```python
from build123d import *

# Parameters (mm, degrees)
F0_W     = 3
F0_H     = 12
F0_W_2   = 7
F0_H_2   = 1
F1_DEPTH = 150
F3_D     = 4.4
F3_DEPTH = 10.4
F3_TIP   = 1.3218933619
F4_SIZE  = 19.99999
F6_DEPTH = 8


# Not quite as in the source:
# - a fillet or chamfer is up to 0.001 mm smaller than in the source, because OpenCascade refuses the exact size


with BuildPart() as f1:
    # F0 (on Front) → F1 (new body)
    with BuildSketch(Plane.XZ):
        with Locations((-8.5, 8)):
            Rectangle(F0_W, F0_H)
        Polygon((-10, 0), (0, 0), (3, 0), (3, 2), (-7, 2), (-10, 2), align=None)
        Polygon((0, -8), (0, 0), (-10, 0), (-10, -10), (0, -10), align=None)
        Polygon((0, -10), (-10, -10), (-10, -11), (10, -11), (10, -10), (3, -10), align=None)
        with Locations((6.5, -9.5)):
            Rectangle(F0_W_2, F0_H_2)
        Polygon((3, -8), (0, -8), (0, -10), (3, -10), (3, -9), align=None)
    extrude(amount=F1_DEPTH)

    # F3
    with Locations(Plane.XY.offset(2)):
        with Locations((-4, -100)):
            Hole(F3_D / 2, depth=F3_DEPTH)
            with Locations((0, 0, -(F3_DEPTH + F3_TIP / 2))):  # 118° drill point
                Cone(0, F3_D / 2, F3_TIP, mode=Mode.SUBTRACT)

    # F4 (size 20 in the source; OpenCascade refuses exactly that, so slightly less here)
    f4_edges = [f1.edges().sort_by_distance(p)[0] for p in [
        (10, -150, -10),
    ]]
    chamfer(f4_edges, length=F4_SIZE)

    # F5 (on face) → F6 (cut, symmetric)
    with BuildSketch(Plane(origin=(0, 0, 0), x_dir=(1, 0, 0), z_dir=(0, 0, -1))):
        with BuildLine():
            ThreePointArc((1.767771953, 138.232238047), (2.3097001843, 139.0432946855), (2.5, 140))
            ThreePointArc((2.5, 140), (-1.767766953, 141.767766953), (0, 137.5))
            Line((0, 137.5), (0, 140.00001))
            Line((0, 140.00001), (1.767771953, 138.232238047))
        make_face()
        with BuildLine():
            Line((0, 140.00001), (0, 137.5))
            ThreePointArc((0, 137.5), (0.9567118473, 137.6903025217), (1.767771953, 138.232238047))
            Line((1.767771953, 138.232238047), (0, 140.00001))
        make_face()
    extrude(amount=F6_DEPTH, both=True, mode=Mode.SUBTRACT)

    # F7: F1 across face


with BuildPart() as f1_1:
    add(f1.part)
    add(f1.part.mirror(Plane(origin=(-4.3205128205, 0, -2.6487179487), x_dir=(1, 0, 0), z_dir=(0, 1, 0))))


solid = f1_1.part
```
Work out the finished part from the listing and answer in its coordinate system (mm). A direction names the side the tool comes from. Give positions to 0.01 mm unless a question says otherwise; leave off trailing zeros. Loops run counter-clockwise (first coordinate to the right, second up) from the corner with the lowest first, then second, coordinate; pieces in that order, holes last. Notation, with made-up numbers: (19.5, 77.5) -> (36.5, 77.5) arc R26 ccw to (36.5, 112.5) -> close; hole circle Ø1 at (80.25, -32.5). An arc over 180 degrees is marked (long way). Write item = value, one per line. Start each with the question number.
(1) Find section B-B on z = -2.5. Give the number of separate pieces and of enclosed holes in the cut face, and give its area (3 significant figures).
(2) Which of the six approach directions +Z, -Z, +X, -X, +Y, -Y give full straight-line access (tool end or side, diameter ignored) to faces 5 (the flat face through (-2, -2, 2)), 6 (the flat face through (-10, -2, 2))?
(3) The mould has two halves that part along Z. Classify faces 1 (the flat face through (0, -2, -4)), 2 (the flat face through (6, -2, -9)), 3 (the flat face through (-4, 144, -3)), 4 (the flat face through (2, -2, -8)): +Z half, -Z half, draft (parallel to the pull), parting line (faces both ways), or undercut.
(4) Find the intervals of material crossed by probe 1 along X at (y, z) = (100, -1); probe 2 along Z at (x, y) = (1.25, 98); probe 3 along Z at (x, y) = (-4.5, 137.5), in increasing order. Write a range as from..to.
(5) Find section A-A on y = -31. Give the vertices of the cut face in (x, z).
(6) Given pin 1 Ø6 at (x, y) = (1.5, 47.5) entering from +Z; pin 2 Ø3.5 at (x, y) = (-4, 100) entering from +Z; pin 3 Ø3 at (x, z) = (-6, -1) entering from +Y, each flat-ended and moving along its own axis, determine where each tip first touches the part or whether it passes through.
(7) Find section C-C on x = 7.5. Give the vertices of the cut face in (y, z).
From the geometry:
q1.separate_pieces = 1
q1.enclosed_holes = 2
q1.area = 2,850 mm^2
q2.face_5 = +Z, +X, +Y, -Y
q2.face_6 = +Z, -Z, -X, +Y, -Y
q3.face_1 = undercut
q3.face_2 = +Z half
q3.face_3 = draft
q3.face_4 = undercut
q4.probe_1 = -10..-6.2, -1.8..0
q4.probe_2 = -11..-8, 0..2
q4.probe_3 = -11..2
q5.outline = (-10, -11) -> (10, -11) -> (10, -9) -> (3, -9) -> (3, -8) -> (0, -8) -> (0, 0) -> (3, 0) -> (3, 2) -> (-7, 2) -> (-7, 14) -> (-10, 14) -> close
q6.pin_1 = 2
q6.pin_2 = -8.67
q6.pin_3 = 147.5
q7.outline = (-132.5, -11) -> (132.5, -11) -> (132.5, -9) -> (-132.5, -9) -> close
